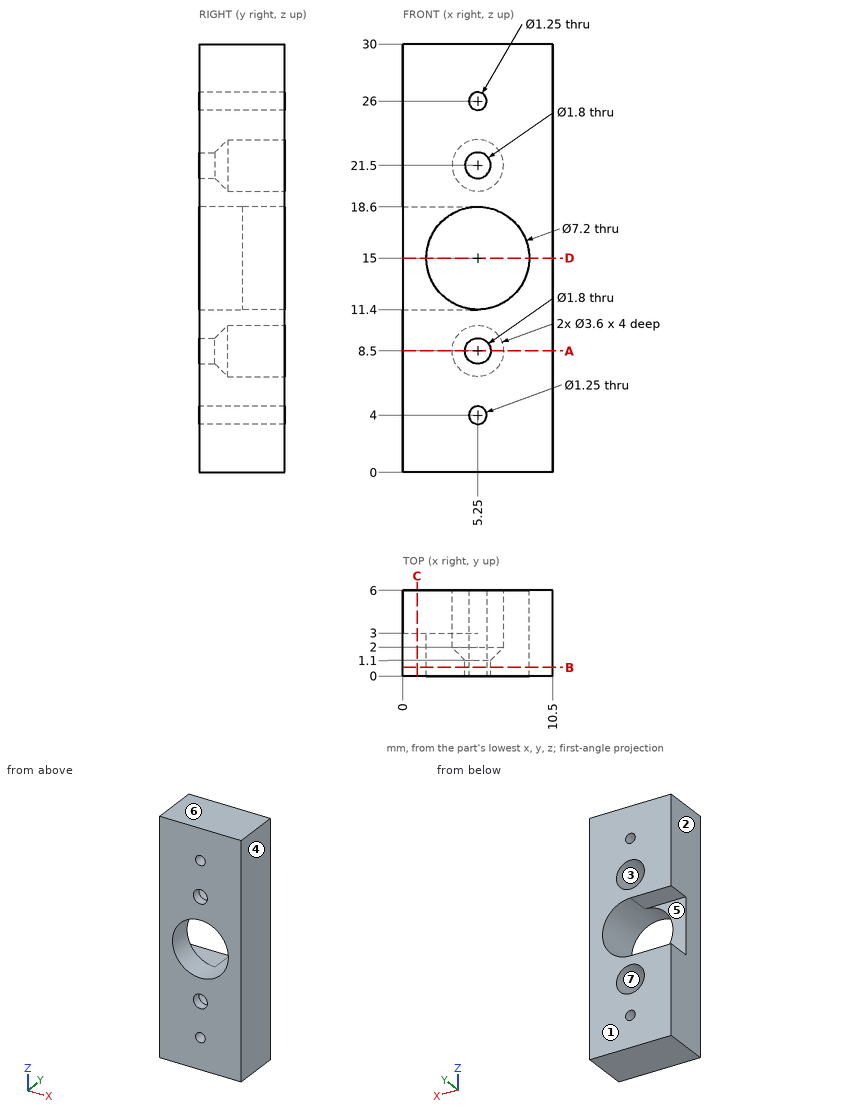
Input: dimensioned drawing with shaded views. Units: mm. Origin: part minimum x, y, z. A direction names the side the tool comes from. Coordinates: 2 decimals unless noted, no trailing zeros. Loops run counter-clockwise (first coordinate to the right, second up) from the corner with the lowest first, then second, coordinate; pieces in that order, holes last. Notation, with made-up numbers: M 44,69 L 73,69 A27 cw 73,102 Z; hole C 84.5,24 d6. An arc over 180 degrees is marked long. Put each result on its own line as item: value.
(1) Cut plane D-D on z = 15. Return the cut outline in (x, y).
Answer sheet:
outline: M 0,0 L 1.65,0 L 1.65,3 L 0,3 Z; M 8.85,0 L 10.5,0 L 10.5,6 L 8.85,6 Z
(2) Cut plane A-A on z = 8.5. Return the cut outline in (x, y), then the cut area to 3 significant figures.
Answer sheet:
outline: M 0,0 L 4.35,0 L 4.35,1.1 L 3.45,2 L 3.45,6 L 0,6 Z; M 6.15,0 L 10.5,0 L 10.5,6 L 7.05,6 L 7.05,2 L 6.15,1.1 Z
area: 44.2 mm^2
(3) Cut plane C-C on x = 1. Return the cut outline in (y, z), then the cut area to 3 significant figures.
Answer sheet:
outline: M 0,0 L 6,0 L 6,11.4 L 3,11.4 L 3,18.6 L 6,18.6 L 6,30 L 0,30 Z
area: 158 mm^2
(4) First-contact query: pin 1 (2 mm diameter, centred on x = 5.25, z = 8.5, fed in from +Y); pin 2 (1.1 mm diameter, centred on x = 5.25, z = 4, fed in from -Y); pin 3 (2.5 mm diameter, centred on x = 2, z = 15, fed in from +Y). Flat tips, straight axial feed; report the tip coordinate or a pass-through.
Answer sheet:
pin 1: stops at y = 1.2
pin 2: passes through
pin 3: stops at y = 3
(5) Material intervals for probe 1 along Z at (x, y) = (5.25, 0.6) (3 decimals); probe 2 along Z at (x, y) = (5.25, 4.7) (3 decimals); probe 3 along X at (y, z) = (4.2, 21.5), sorted ascending.
Answer sheet:
probe 1: z = 0 to 3.375, 4.625 to 7.6, 9.4 to 11.4, 18.6 to 20.6, 22.4 to 25.375, 26.625 to 30
probe 2: z = 0 to 3.375, 4.625 to 6.7, 10.3 to 11.4, 18.6 to 19.7, 23.3 to 25.375, 26.625 to 30
probe 3: x = 0 to 3.45, 7.05 to 10.5
(6) Access query for the marked faces 5, 6 and 7. Directions: +Z, -Z, +X, -X, +Y, -Y. A direction counts if a zero-diameter tool reaches every point of the face in a straight line with its end or side. Return the directions, or none.
Answer sheet:
face 5: -X, +Y
face 6: +Z, +X, -X, +Y, -Y
face 7: +Y
(7) Cut plane B-B on y = 0.6. Return the cut outline in (x, z) (3 decimals), then the cut area to 3 significant figures.
Answer sheet:
outline: M 0,0 L 10.5,0 L 10.5,30 L 0,30 Z; hole C 5.25,15 d7.2; hole C 5.25,8.5 d1.8; hole C 5.25,21.5 d1.8; hole C 5.25,4 d1.25; hole C 5.25,26 d1.25
area: 267 mm^2
(8) Draft query along X for the marked faces 1, 2, 3 and 4. Return one class per face: pulls with the +X half, pulls with the -X half, needs draft (parallel to the pull), parting line crosses it, or undercut.
Answer sheet:
face 1: needs draft
face 2: pulls with the -X half
face 3: undercut
face 4: pulls with the +X half
